Design review of the part built by this model. Coordinates are the model's own, in mm. Face numbers are marked on the shaded views. A direction names the side the tool comes from. Give positions to 0.01 mm unless a question says otherwise; leave off trailing zeros. Order: outer loops, then holes, each group sorted by start corner. A loop starts at its lowest first (then second) coordinate and runs counter-clockwise, first axis right, second up. Notation, with made-up numbers: (-36, 83.25) -> (-3, 83.25) arc R18 ccw to (-3, 106.25) -> close; hole circle Ø3 at (31.5, -20). An arc over 180 degrees is marked (long way). One line per item, written item: value.
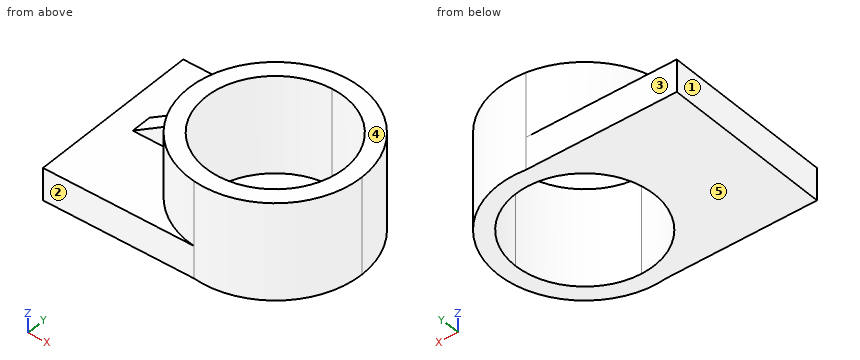
from build123d import *

# Parameters (mm, degrees)
F1_DEPTH = 12.7
F2_DEPTH = 38.1
F3_W     = 19.9459594991
F3_H     = 7.9969605431
F4_DEPTH = 12.7
F6_DEPTH = 25.4


with BuildPart() as f1:
    # F0 (on Top) → F1 (new body)
    with BuildSketch(Plane.XY):
        with BuildLine():
            Line((10.3908990951, 36.1372716725), (-48.721820116, 36.1372716725))
            Line((-48.721820116, 36.1372716725), (-48.721820116, -31.0572721064))
            Line((-48.721820116, -31.0572721064), (10.3908990951, -31.0572721064))
            ThreePointArc((10.3908990951, -31.0572721064), (-19.1043346565, 2.539999783), (10.3908990951, 36.1372716725))
        make_face()
    extrude(amount=F1_DEPTH)

    # F0 (on Top) → F2 (join)
    with BuildSketch(Plane.XY):
        with BuildLine():
            ThreePointArc((48.6606984776, 2.539999783), (37.1318476752, 28.0024929013), (10.3908990951, 36.1372716725))
            Line((10.3908990951, 36.1372716725), (14.7781819105, 36.1372716725))
            Line((14.7781819105, 36.1372716725), (14.7781819105, 29.7147905973))
            ThreePointArc((14.7781819105, 29.7147905973), (33.9936607726, 21.7554786451), (41.9529727248, 2.539999783))
            ThreePointArc((41.9529727248, 2.539999783), (33.9936607726, -16.675479079), (14.7781819105, -24.6347910312))
            Line((14.7781819105, -24.6347910312), (14.7781819105, -31.0572721064))
            Line((14.7781819105, -31.0572721064), (10.3908990951, -31.0572721064))
            ThreePointArc((10.3908990951, -31.0572721064), (37.1318476752, -22.9224933352), (48.6606984776, 2.539999783))
        make_face()
        with BuildLine():
            Line((14.7781819105, 36.1372716725), (10.3908990951, 36.1372716725))
            ThreePointArc((10.3908990951, 36.1372716725), (-19.1043346565, 2.539999783), (10.3908990951, -31.0572721064))
            Line((10.3908990951, -31.0572721064), (14.7781819105, -31.0572721064))
            Line((14.7781819105, -31.0572721064), (14.7781819105, -24.6347910312))
            ThreePointArc((14.7781819105, -24.6347910312), (-12.3966089037, 2.539999783), (14.7781819105, 29.7147905973))
            Line((14.7781819105, 29.7147905973), (14.7781819105, 36.1372716725))
        make_face()
    extrude(amount=F2_DEPTH)

    # F3 (on face) → F4 (join)
    with BuildSketch(Plane.XY.offset(12.7)):
        with Locations((-28.9819748448, 3.9984802715)):
            Rectangle(F3_W, F3_H)
    extrude(amount=F4_DEPTH)

    # F5 (on face) → F6 (cut)
    with BuildSketch(Plane.XZ):
        Polygon((-38.9549545944, 12.7), (-19.0089950952, 25.4), (-38.9549545944, 25.4), align=None)
    extrude(amount=-F6_DEPTH, mode=Mode.SUBTRACT)


solid = f1.part
Item 1: Add section D-D on x = -21. Give the boundary of the cut face in (y, z), plus the area to 3 significant figures.
Returned:
outline: (-31.06, 0) -> (36.14, 0) -> (36.14, 12.7) -> (8, 12.7) -> (8, 24.13) -> (0, 24.13) -> (0, 12.7) -> (-31.06, 12.7) -> close
area: 945 mm²
Item 2: Add section B-B on x = 35. Give the boundary of the cut face in (y, z), plus the area to 3 significant figures.
Returned:
outline: (-24.65, 0) -> (-15.61, 0) -> (-15.61, 38.1) -> (-24.65, 38.1) -> close; (20.69, 0) -> (29.73, 0) -> (29.73, 38.1) -> (20.69, 38.1) -> close
area: 688 mm²
Item 3: Machinability: for the marked faces 1 and 2, which of the approach directions +Z, -Z, +X, -X, +Y, -Y give a long, thin tool a straight path to every point of the face, cutting with its end or side? Answer none if there is none.
Returned:
face 1: +Z, -Z, -X, +Y, -Y
face 2: +Z, -Z, -X, -Y
Item 4: Clearance check with flat-ended pins moving along their axes: P1, Ø6, axis at x = 6, z = 33, coming from the +Y side; P2, Ø6, axis at y = 9, z = 26, coming from the +X side; P3, Ø6.5, axis at x = -33, z = 18.5, coming from the -Y side; P4, Ø12, axis at x = 25.5, y = 15, coming from the +Z side. State where each tip first meets the part, or that it passes through.
Returned:
P1: y = 35.93
P2: x = 48.48
P3: y = 0
P4: through
Item 5: Draft analysis for pull direction Z (two halves, no side actions). For the marked faces 3, 4 and 5, state which applies: pulls with the +Z half, pulls with the -Z half, needs draft (parallel to the pull), parting line crosses it, or undercut.
Returned:
face 3: needs draft
face 4: pulls with the +Z half
face 5: pulls with the -Z half
Item 6: To check wall thickness, follow line 1 along X through (y, z) = (2.5, 36.5); line 2 along Z through (x, y) = (-23, -2); line 3 along Y through (x, z) = (2, 7.5). State the ranges of each line that lie inside material, in increasing order. Write a range as from..to.
Returned:
line 1: -19.1..-12.4, 41.95..48.66
line 2: 0..12.7
line 3: -31.06..-21.44, 26.52..36.14
Item 7: Add section A-A on z = 11.5. Give the boundary of the cut face in (x, y).
Returned:
outline: (-48.72, -31.06) -> (10.39, -31.06) arc R33.88 ccw (long way) to (10.39, 36.14) -> (-48.72, 36.14) -> close; hole circle Ø54.35 at (14.78, 2.54)
Item 8: Add section C-C on y = 11.5. Give the boundary of the cut face in (x, z), plus the area to 3 significant figures.
Returned:
outline: (-48.72, 0) -> (-10.88, 0) -> (-10.88, 38.1) -> (-17.9, 38.1) -> (-17.9, 12.7) -> (-48.72, 12.7) -> close; (40.43, 0) -> (47.45, 0) -> (47.45, 38.1) -> (40.43, 38.1) -> close
area: 926 mm²
